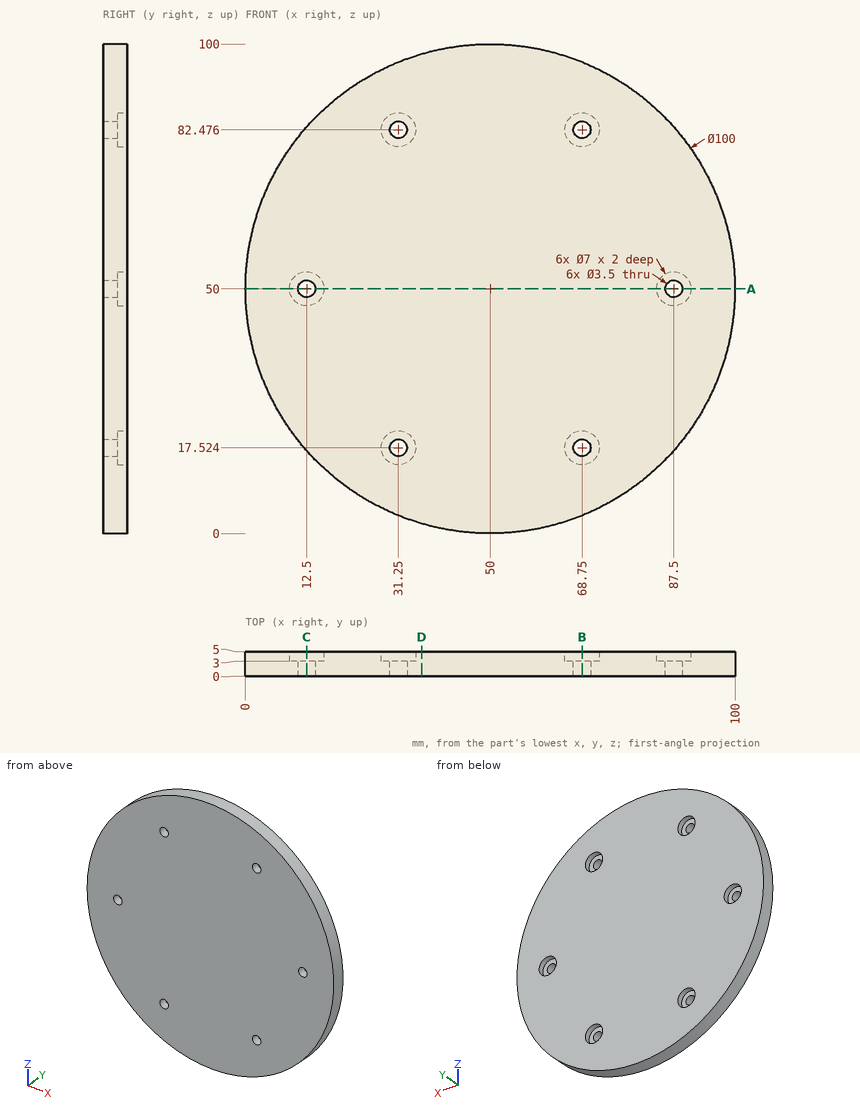
Here's the drawing with two shaded views (mm, measured from the low corner). I have some questions. Give positions to 0.01 mm unless a question says otherwise; leave off trailing zeros. Order: outer loops, then holes, each group sorted by start corner. A loop starts at its lowest first (then second) coordinate and runs counter-clockwise, first axis right, second up. Notation, with made-up numbers: (-11, 50) - (44, 50) arc R31 cw to (44, 83) - close; hole circle Ø10 at (-14.5, 24.5). An arc over 180 degrees is marked (long way). Use a Markdown table: item, result. Add a question column.
Q1. If we section it at B-B on x = 68.75: Write out the boundary of the cut face in (y, z), plus the area to 3 significant figures.
Q2. If we section it at C-C on x = 12.5: Write out the boundary of the cut face in (y, z).
Q3. If we section it at D-D on x = 36: Write out the boundary of the cut face in (y, z), plus the area to 3 significant figures.
Q4. If we section it at A-A on z = 50: Write out the boundary of the cut face in (x, y).
Q5. I'm going to push flat-ended pins straight in: pin 1 (5.5 mm diameter, centred on x = 68.75, z = 82.476, fed in from +Y); pin 2 (2 mm diameter, centred on x = 87.5, z = 50, fed in from +Y); pin 3 (3 mm diameter, centred on x = 28, y = 1.5, fed in from +Z). Where does each tip first touch, or does it pass through?
Q6. Please list where these lines run through material, in increasing order: line 1 along Z through (x, y) = (68.75, 3.75); line 2 along X through (y, z) = (2.65, 83); line 3 along Z through (x, y) = (31.25, 1.3).
Answers follow:
| question | item | result |
|---|---|---|
| 1 | outline | (0, 3.65) - (5, 3.65) - (5, 14.02) - (3, 14.02) - (3, 15.77) - (0, 15.77) - close; (0, 19.27) - (3, 19.27) - (3, 21.02) - (5, 21.02) - (5, 78.98) - (3, 78.98) - (3, 80.73) - (0, 80.73) - close; (0, 84.23) - (3, 84.23) - (3, 85.98) - (5, 85.98) - (5, 96.35) - (0, 96.35) - close |
| 1 | area | 415 mm^2 |
| 2 | outline | (0, 16.93) - (5, 16.93) - (5, 46.5) - (3, 46.5) - (3, 48.25) - (0, 48.25) - close; (0, 51.75) - (3, 51.75) - (3, 53.5) - (5, 53.5) - (5, 83.07) - (0, 83.07) - close |
| 3 | outline | (0, 2) - (5, 2) - (5, 98) - (0, 98) - close |
| 3 | area | 480 mm^2 |
| 4 | outline | (0, 0) - (10.75, 0) - (10.75, 3) - (9, 3) - (9, 5) - (0, 5) - close; (14.25, 0) - (85.75, 0) - (85.75, 3) - (84, 3) - (84, 5) - (16, 5) - (16, 3) - (14.25, 3) - close; (89.25, 0) - (100, 0) - (100, 5) - (91, 5) - (91, 3) - (89.25, 3) - close |
| 5 | pin 1 | stops at y = 3 |
| 5 | pin 2 | passes through |
| 5 | pin 3 | stops at z = 95.6 |
| 6 | line 1 | z = 3.65 to 14.02, 21.02 to 78.98, 85.98 to 96.35 |
| 6 | line 2 | x = 12.44 to 29.58, 32.92 to 67.08, 70.42 to 87.56 |
| 6 | line 3 | z = 3.65 to 15.77, 19.27 to 80.73, 84.23 to 96.35 |
